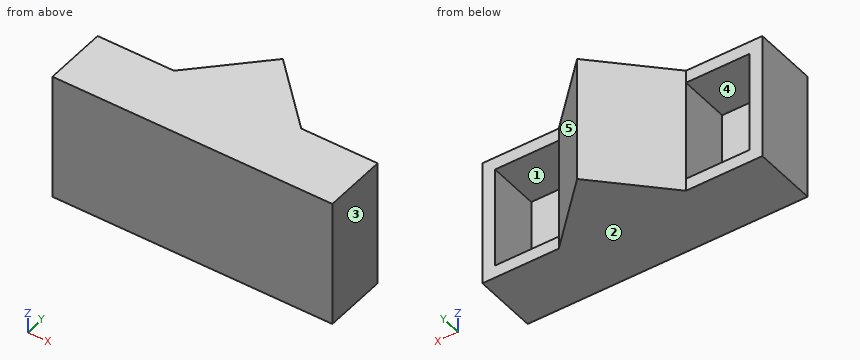
```python
from build123d import *

# Parameters (mm, degrees)
BOSS_EXTRUDE1_DEPTH = 100
BOSS_EXTRUDE2_DEPTH = 50
SKETCH5_W           = 100
SKETCH5_H           = 50
BOSS_EXTRUDE3_DEPTH = 10


with BuildPart() as part:
    # Sketch2 → Boss-Extrude1 (new body)
    with BuildSketch(Plane.XY):
        Polygon((-50, 0), (50, 0), (50, 50), (0, 100), (-50, 50), align=None)
    extrude(amount=BOSS_EXTRUDE1_DEPTH)

    # Sketch4 → Boss-Extrude2 (add)
    with BuildSketch(Plane(origin=(50, 0, 0), x_dir=(0, 0, -1), z_dir=(1, 0, 0))):
        Polygon((-100, 50), (-100, 0), (0, 0), (0, 50), (-10, 50), (-10, 10), (-90, 10), (-90, 50), align=None)
    boss_extrude2 = extrude(amount=BOSS_EXTRUDE2_DEPTH)

    # Sketch5 → Boss-Extrude3 (add)
    with BuildSketch(Plane(origin=(100, 0, 0), x_dir=(0, 0, -1), z_dir=(1, 0, 0))):
        with Locations((-50, 25)):
            Rectangle(SKETCH5_W, SKETCH5_H)
    boss_extrude3 = extrude(amount=BOSS_EXTRUDE3_DEPTH)

    # Mirror1: Boss-Extrude2, Boss-Extrude3 across plane
    add(boss_extrude2.mirror(Plane(origin=(0, 0, 0), x_dir=(0, 0, 1), z_dir=(1, 0, 0))))
    add(boss_extrude3.mirror(Plane(origin=(0, 0, 0), x_dir=(0, 0, 1), z_dir=(1, 0, 0))))


solid = part.part
```
Can you work these out from the model? Positions are in its coordinate system, mm. Face numbers are marked on the shaded views. A direction names the side the tool comes from. Coordinates: 2 decimals unless noted, no trailing zeros. Write each loop counter-clockwise with the first axis right and the second up, starting at its lowest first coordinate (ties: lowest second). Pieces come first, ordered by that corner, then holes. Notation, with made-up numbers: M -22,-8 L 26,-8 A12 cw 26,5 Z; hole C -24.75,-13.5 d8. An arc over 180 degrees is marked long. Answer as CSV lines item,"result".
Item 1: I'm going to push flat-ended pins straight in: P1, Ø1, axis at x = 12, z = 38, coming from the +Y side; P2, Ø25, axis at x = -84.5, z = 41.5, coming from the +Y side; P3, Ø1, axis at y = 73, z = 39, coming from the -X side. Where does each tip first touch, or does it pass through?
Geometry results:
P1,"stops at y = 88.5"
P2,"stops at y = 10"
P3,"stops at x = -27.5"
Item 2: We'd pull the mould along Z, two halves only. Please class the marked faces 1, 2 and 3: +Z half, -Z half, draft (parallel to the pull), parting line (faces both ways), or undercut.
Geometry results:
face 1,"undercut"
face 2,"-Z half"
face 3,"draft"
Item 3: Imagine slicing it at D-D on y = 73. List the corners of the cut face in (x, z) for me, plus the area to 3 significant figures.
Geometry results:
outline,"M -27,0 L 27,0 L 27,100 L -27,100 Z"
area,"5,400 mm2"
Item 4: On a 3-axis mill with a long thin cutter (end or side, diameter ignored), from which of +Z, -Z, +X, -X, +Y, -Y can I reach the whole of each face in a straight line? I mean the marked faces 4 and 5. Say none if no direction works.
Geometry results:
face 4,"+Y"
face 5,"+Z, -Z, +X, +Y"
Item 5: Please list where these lines run through material, in increasing order: line 1 along X through (y, z) = (15, 78); line 2 along Z through (x, y) = (-97.5, 13); line 3 along Y through (x, z) = (76, 13).
Geometry results:
line 1,"x = -110 to -100, -50 to 50, 100 to 110"
line 2,"z = 0 to 10, 90 to 100"
line 3,"y = 0 to 10"
Item 6: Imagine slicing it at A-A on y = 22. List the corners of the cut face in (x, z) for me, plus the area to 3 significant figures.
Geometry results:
outline,"M -110,0 L 110,0 L 110,100 L -110,100 Z; hole M -100,10 L -50,10 L -50,90 L -100,90 Z; hole M 50,10 L 100,10 L 100,90 L 50,90 Z"
area,"14,000 mm2"
Item 7: Imagine slicing it at B-B on z = 7.5. List the corners of the cut face in (x, y) for me.
Geometry results:
outline,"M -110,0 L 110,0 L 110,50 L 50,50 L 0,100 L -50,50 L -110,50 Z"
Item 8: Imagine slicing it at C-C on x = 83. List the corners of the cut face in (y, z) for me.
Geometry results:
outline,"M 0,0 L 50,0 L 50,10 L 10,10 L 10,90 L 50,90 L 50,100 L 0,100 Z"
